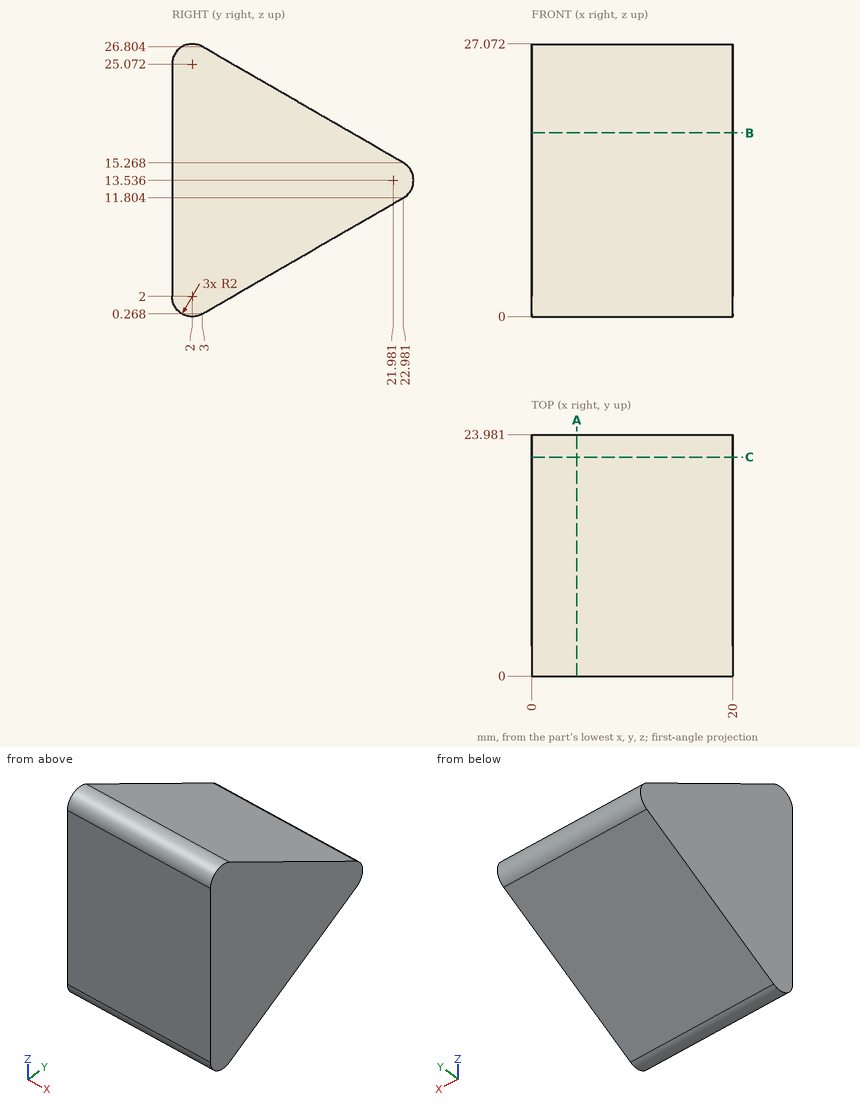
Source: three-view drawing plus pictorial views. Frame: mm from the lowest corner of the part. Round coordinates to 2 decimals unless told otherwise and drop trailing zeros. Loops run counter-clockwise (first coordinate to the right, second up) from the corner with the lowest first, then second, coordinate; pieces in that order, holes last.
1. Section query B-B on z = 18.25. Output: boundary loops of the cut face in (x, y).
2. Section query A-A on x = 4.5. Output: boundary loops of the cut face in (y, z).
3. Section query C-C on y = 21.75. Output: boundary loops of the cut face in (x, z), and give its area (3 significant figures).
4. Ray query, L1, parallel to Z at x = 12, y = 10.25; L2, parallel to Y at x = 6.5, z = 7.5 (1 decimal); L3, parallel to Y at x = 7.5, z = 16.5 (1 decimal). Return the intervals inside material, ascending.
5. Contact query for flat-ended pins moving along their axis: pin 1 (12 mm diameter, centred on y = 20, z = 3, fed in from -X); pin 2 (12 mm diameter, centred on x = 9, y = 15.5, fed in from -Z); pin 3 (1.5 mm diameter, centred on x = 13.5, y = 4, fed in from -Z); pin 4 (8 mm diameter, centred on x = 16.5, y = 16, fed in from +Z). Output: stop coordinate, or through.
Answers below:
1. outline: (0, 0) - (20, 0) - (20, 17.82) - (0, 17.82) - close
2. outline: (0, 2) arc R2 ccw to (3, 0.27) - (22.98, 11.8) arc R2 ccw to (22.98, 15.27) - (3, 26.8) arc R2 ccw to (0, 25.07) - close
3. outline: (0, 11.09) - (20, 11.09) - (20, 15.98) - (0, 15.98) - close
3. area: 97.7 mm2
4. L1: z = 4.45 to 22.62
4. L2: y = 0 to 15.5
4. L3: y = 0 to 20.8
5. pin 1: passes through
5. pin 2: stops at z = 4.02
5. pin 3: stops at z = 0.41
5. pin 4: stops at z = 21.61
